```python
from build123d import *

# Parameters (mm, degrees)
SKETCH1_R           = 4.7625
BOSS_EXTRUDE1_DEPTH = 14.478
SKETCH2_W           = 9.525
SKETCH2_H           = 1.905
CUT_EXTRUDE1_DEPTH  = 3.175
SKETCH3_R           = 1.999996
CUT_EXTRUDE2_DEPTH  = 5


with BuildPart() as part:
    # Sketch1 → Boss-Extrude1 (new body)
    with BuildSketch(Plane(origin=(0, 0, 0), x_dir=(1, 0, 0), z_dir=(0, 1, 0))):
        with Locations(Location((0, 0, 0), (0, 0, 270))):
            Circle(SKETCH1_R)
    extrude(amount=-BOSS_EXTRUDE1_DEPTH)

    # Sketch2 → Cut-Extrude1 (cut)
    with BuildSketch(Plane(origin=(0, 0, 0), x_dir=(1, 0, 0), z_dir=(0, 1, 0))):
        Rectangle(SKETCH2_W, SKETCH2_H)
    extrude(amount=-CUT_EXTRUDE1_DEPTH, mode=Mode.SUBTRACT)

    # Sketch3 → Cut-Extrude2 (cut)
    with BuildSketch(Plane.XZ.offset(14.478)):
        with Locations(Location((0, 0, 0), (0, 0, 270))):
            Circle(SKETCH3_R)
    extrude(amount=-CUT_EXTRUDE2_DEPTH, mode=Mode.SUBTRACT)


solid = part.part
```
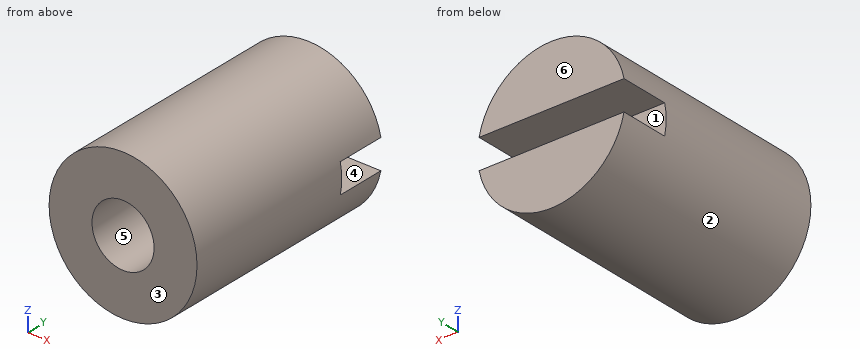
CAD build for the part. Positions are in the model's coordinates, mm. Face numbers are marked on the shaded views. A direction names the side the tool comes from. Round coordinates to 2 decimals unless told otherwise and drop trailing zeros. Order: outer loops, then holes, each group sorted by start corner. A loop starts at its lowest first (then second) coordinate and runs counter-clockwise, first axis right, second up. Notation, with made-up numbers: (-33.75, 89.25) - (10.25, 89.25) arc R14 ccw to (10.25, 103.25) - close; hole circle Ø1 at (76.5, 49). An arc over 180 degrees is marked (long way). Answer in a Markdown table with one row per item. Add a question column.
(1) Drop flat-ended pins along their axis: pin 1 Ø5 at (y, z) = (-11.5, -3.5) entering from -X; pin 2 Ø1.6 at (x, y) = (-1, -2) entering from -Z; pin 3 Ø1.2 at (x, z) = (1, -0.5) entering from -Y. Give the stop position or say it passes through.
(2) Band-saw the part on B-B on z = 0. List the corners of the cut face in (x, y) (1 decimal).
(3) Mould opens along Z. For the marked faces 1, 2 and 3 say: +Z half, -Z half, draft (parallel to the pull), parting line (faces both ways), or undercut.
(4) Band-saw the part on A-A on x = 0. List the corners of the cut face in (y, z) (1 decimal).
(5) Band-saw the part on C-C on y = -12.25. List the corners of the cut face in (x, z) (1 decimal).
(6) Band-saw the part on D-D on y = -6.5. List the corners of the cut face in (x, z) (1 decimal), and give its area (3 significant figures).
(7) 3-axis set-ups, long thin cutter, end or side, ignore diameter. For the marked faces 4, 5 and 6: which of +Z, -Z, +X, -X, +Y, -Y reach the whole face in a straight line?
(8) Probe L1, parallel to X at y = -12.75, z = 0; L2, parallel to Y at x = -2.75, z = -0.5 (3 decimals); L3, parallel to Z at x = 1.75, y = -3. List the from-to ranges inside material, lowest first. Write a range as [from, to].
Data:
| question | item | result |
|---|---|---|
| 1 | pin 1 | stops at x = -4.66 |
| 1 | pin 2 | stops at z = -4.76 |
| 1 | pin 3 | stops at y = -9.48 |
| 2 | outline | (-4.8, -14.5) - (-2, -14.5) - (-2, -9.5) - (2, -9.5) - (2, -14.5) - (4.8, -14.5) - (4.8, -3.2) - (-4.8, -3.2) - close |
| 3 | face 1 | undercut |
| 3 | face 2 | parting line |
| 3 | face 3 | draft |
| 4 | outline | (-14.5, -4.8) - (0, -4.8) - (0, -1) - (-3.2, -1) - (-3.2, 1) - (0, 1) - (0, 4.8) - (-14.5, 4.8) - (-14.5, 2) - (-9.5, 2) - (-9.5, -2) - (-14.5, -2) - close |
| 5 | outline | circle Ø9.5 at (0, 0); hole circle Ø4 at (0, 0) |
| 6 | outline | circle Ø9.5 at (0, 0) |
| 6 | area | 71.3 mm^2 |
| 7 | face 4 | +X, -X, +Y |
| 7 | face 5 | -Y |
| 7 | face 6 | +Z, -Z, +X, -X, +Y |
| 8 | L1 | x = [-4.76, -2], [2, 4.76] |
| 8 | L2 | y = [-14.478, -3.175] |
| 8 | L3 | z = [-4.43, -0.95], [0.95, 4.43] |
